from build123d import *

# Parameters (mm, degrees)
SKETCH1_R           = 5
SKETCH1_R_2         = 1.8
BOSS_EXTRUDE1_DEPTH = 10
SKETCH3_R           = 11.025
CUT_EXTRUDE2_DEPTH  = 7.025
SKETCH4_R           = 12.525
CUT_EXTRUDE3_DEPTH  = 1.425
CHAMFER1_SIZE       = 0.5
SKETCH5_R           = 1.8
CUT_EXTRUDE4_DEPTH  = 10
CHAMFER2_SIZE       = 0.5


with BuildPart() as part:
    # Sketch1 → Boss-Extrude1 (new body)
    with BuildSketch(Plane.XY):
        with BuildLine():
            Line((-40.746699048, 8.183561953), (-33.214821075, -10))
            Line((-33.214821075, -10), (-9.797958971, -10))
            ThreePointArc((-9.797958971, -10), (0, -14), (9.797958971, -10))
            Line((9.797958971, -10), (19.5, -10))
            Line((19.5, -10), (19.5, -3.981225471))
            ThreePointArc((19.5, -3.981225471), (20, 4.0125), (20.5, -3.981225471))
            Line((20.5, -3.981225471), (20.5, -10))
            Line((20.5, -10), (33.214821075, -10))
            Line((33.214821075, -10), (40.746699048, 8.183561953))
            ThreePointArc((40.746699048, 8.183561953), (0, 18.25), (-40.746699048, 8.183561953))
        make_face()
        Circle(SKETCH1_R, mode=Mode.SUBTRACT)
        with Locations((-32.07645249, 8.189406634)):
            Circle(SKETCH1_R_2, mode=Mode.SUBTRACT)
        with Locations(Location((32.07645249, 8.189406634, 0), (0, 0, 180))):
            Circle(SKETCH1_R_2, mode=Mode.SUBTRACT)
        Polygon((-25.988511975, 6.5901118), (-35.250404289, 2.75371039), (-31.414002879, -6.508181923), (-22.152110566, -2.671780514), align=None, mode=Mode.SUBTRACT)
    extrude(amount=BOSS_EXTRUDE1_DEPTH)

    # Sketch3 → Cut-Extrude2 (cut)
    with BuildSketch(Plane(origin=(0, 0, 0), x_dir=(-1, 0, 0), z_dir=(0, 0, -1))):
        Circle(SKETCH3_R)
    extrude(amount=-CUT_EXTRUDE2_DEPTH, mode=Mode.SUBTRACT)

    # Sketch4 → Cut-Extrude3 (cut)
    with BuildSketch(Plane(origin=(0, 0, 0), x_dir=(-1, 0, 0), z_dir=(0, 0, -1))):
        Circle(SKETCH4_R)
    extrude(amount=-CUT_EXTRUDE3_DEPTH, mode=Mode.SUBTRACT)

    # Chamfer1
    chamfer1_edges = [part.edges().sort_by_distance(p)[0] for p in [
        (20, 4.0125, 10),
        (-24.070311271, 1.959165643, 10),
        (-30.619458132, 4.671911095, 10),
        (-33.332203584, -1.877235766, 10),
        (-26.783056723, -4.589981218, 10),
    ]]
    chamfer(chamfer1_edges, length=CHAMFER1_SIZE)

    # Sketch5 → Cut-Extrude4 (cut)
    with BuildSketch(Plane(origin=(-29.114518455, -12.059628406, 0), x_dir=(0, 0, -1), z_dir=(0.923879532511288, 0.3826834323650871, 0))):
        with Locations(Location((-4.75, 11.018842374, 0), (0, 0, 90))):
            Circle(SKETCH5_R)
    extrude(amount=-CUT_EXTRUDE4_DEPTH, mode=Mode.SUBTRACT)

    # Chamfer2
    chamfer2_edges = [part.edges().sort_by_distance(p)[0] for p in [
        (-36.980760062, -0.908219024, 10),
        (-21.506390023, -10, 10),
        (0, -14, 10),
        (14.648979486, -10, 10),
        (26.857410538, -10, 10),
        (36.980760062, -0.908219024, 10),
        (0, 18.25, 10),
    ]]
    chamfer(chamfer2_edges, length=CHAMFER2_SIZE)


solid = part.part
Input: part model. Units: mm. Frame: model coordinates. A direction names the side the tool comes from. Give positions to 0.01 mm unless a question says otherwise; leave off trailing zeros. Order: outer loops, then holes, each group sorted by start corner. A loop starts at its lowest first (then second) coordinate and runs counter-clockwise, first axis right, second up.
Q1. Set-up query: faces 4 (the flat face through (-30.55, 4.7, 4.68)), 5 (the flat face through (-5, -2, 7.025)), 6 (the flat face through (27, -10, 5)). Return all of +Z, -Z, +X, -X, +Y, -Y with unobstructed straight access to the full face (end or side cutting, diameter ignored); none if empty.
Checked values:
face 4: +Z, -Z
face 5: -Z
face 6: +Z, -Z, +X, -Y
Q2. Section A-A on x = 0. Output: boundary loops of the cut face in (y, z) (3 decimals).
Checked values:
outline: (-14, 0) - (-12.525, 0) - (-12.525, 1.425) - (-11.025, 1.425) - (-11.025, 7.025) - (-5, 7.025) - (-5, 10) - (-13.5, 10) - (-14, 9.5) - close; (5, 7.025) - (11.025, 7.025) - (11.025, 1.425) - (12.525, 1.425) - (12.525, 0) - (18.25, 0) - (18.25, 9.5) - (17.75, 10) - (5, 10) - close
Q3. Section B-B on z = 7.75. State how many separate pieces and enclosed holes the cut face has, and give its area (3 significant figures).
Checked values:
separate pieces: 1
enclosed holes: 4
area: 1,700 mm2
Q4. Ray query, probe 1 along Y at (x, z) = (-0.5, 6); probe 2 along X at (y, z) = (-2.5, 3.25); probe 3 along X at (y, z) = (5.5, 6). Return the intervals inside material, ascending.
Checked values:
probe 1: y = -13.99 to -11.01, 11.01 to 18.25
probe 2: x = -22.22 to -10.74, 10.74 to 16.86, 23.14 to 36.32
probe 3: x = -39.64 to -28.62, -25.54 to -9.56, 9.56 to 39.64
Q5. Draft query along X for faces 1 (the flat face through (36.7, -0.94, 9.75)), 2 (the flat face through (-23.81, 1.98, 9.75)), 3 (the conical face through (0.59, 17.89, 9.86)). Return one class per face: +X half, -X half, draft (parallel to the pull), parting line (faces both ways), or undercut.
Checked values:
face 1: +X half
face 2: undercut
face 3: parting line
Q6. Contact query for flat-ended pins moving along their axis: pin 1 Ø1.8 at (y, z) = (-6.5, 4.5) entering from +X; pin 2 Ø3 at (x, z) = (-27, 5) entering from +Y; pin 3 Ø3 at (y, z) = (7, 6.5) entering from +X; pin 4 Ø3 at (x, y) = (32.08, 8.19) entering from -Z. Output: stop coordinate, or through.
Checked values:
pin 1: stops at x = 35.04
pin 2: stops at y = 14.45
pin 3: stops at x = 40.75
pin 4: passes through
